Work out the finished part from the listing and answer in its coordinate system (mm). A direction names the side the tool comes from. Coordinates: 2 decimals unless noted, no trailing zeros. Order: outer loops, then holes, each group sorted by start corner. A loop starts at its lowest first (then second) coordinate and runs counter-clockwise, first axis right, second up. Notation, with made-up numbers: M 14,-11.5 L 29,-11.5 A15 cw 29,-6.5 Z; hole C -8.75,37.5 d4. An arc over 180 degrees is marked long. Write item = value, one per line. Start each with the question number.
Q1. Find section B-B on x = 20. Give the vertices of the cut face in (y, z), and give its area (3 significant figures).
Q2. A tool of negligible diameter and unlimited length cuts with its end or side. For faces 1 (the flat face through (-45.422, -23, 29)), 2 (the cylindrical face through (17.07, 13.09, 30.12)), from which of +Z, -Z, +X, -X, +Y, -Y can it reach the whole face along a straight path? Write none if from no direction.
Q3. Each of these flat-tipped pins is pushed along its axis until it touches: P1, Ø4, axis at x = -23.5, z = 32, coming from the +Y side; P2, Ø16.5, axis at x = 0, y = 0, coming from the +Z side; P3, Ø6, axis at y = -0.5, z = 34.5, coming from the -X side. Where does it stop, or does it pass through?
Q4. Straight lines are drawn through the part: line 1 along Y through (x, z) = (0, 1); line 2 along Y through (x, z) = (0, 15.5); line 3 along Z through (x, y) = (-19, -7.5). For each, find the intervals that lie inside material, in ascending order.
Q5. Find section C-C on x = -8. Give the vertices of the cut face in (y, z), and give its area (3 significant figures).
Q6. Determine the mould class of faces 3 (the flat face through (45.422, -23, 29)), 4 (the flat face through (-1, -24.666, 29)), 5 (the flat face through (-4, 4, 3)) for opening direction X: released by +X, released by -X, zero draft, split by the parting line, or undercut.
Q7. Find section A-A on y = 3.5. Give the vertices of the cut face in (x, z), and give its area (3 significant figures).
```python
from build123d import *

# Parameters (mm, degrees)
SKETCH1_R           = 24.241475666
SKETCH1_R_2         = 21.51
BOSS_EXTRUDE1_DEPTH = 58
SKETCH1_4_R         = 21.51
BOSS_EXTRUDE2_DEPTH = 3


with BuildPart() as part:
    # Sketch1 → Boss-Extrude1 (new body)
    # profile 1 of 2: a face of its own
    with BuildSketch(Plane.XY):
        Circle(SKETCH1_R)
        with Locations(Location((0, 0, 0), (0, 0, 180))):
            Circle(SKETCH1_R_2, mode=Mode.SUBTRACT)
    # profile 2 of 2: a face of its own
    with BuildSketch(Plane.XY):
        with BuildLine():
            Line((-45.421940828, -20.666245921), (-45.421940828, -24.666245921))
            Line((-45.421940828, -24.666245921), (45.421940828, -24.666245921))
            Line((45.421940828, -24.666245921), (45.421940828, -20.666245921))
            add(Edge.make_bspline(
                [(45.421940828, -20.666245921), (21.532203305, -20.666245921), (24.241475666, -19.078845964), (24.241475666, 0)],
                knots=[0, 0, 0, 0, 1, 1, 1, 1], degree=3))
            ThreePointArc((24.241475666, 0), (0, -24.241475666), (-24.241475666, 0))
            add(Edge.make_bspline(
                [(-45.421940828, -20.666245921), (-21.532203305, -20.666245921), (-24.241475666, -19.078845964), (-24.241475666, 0)],
                knots=[0, 0, 0, 0, 1, 1, 1, 1], degree=3))
        make_face()
    extrude(amount=BOSS_EXTRUDE1_DEPTH)

    # Sketch1_4 → Boss-Extrude2 (add)
    with BuildSketch(Plane.XY):
        with Locations(Location((0, 0, 0), (0, 0, 180))):
            Circle(SKETCH1_4_R)
        with BuildLine():
            ThreePointArc((0, -5.15), (-3.641599923, 3.641599923), (5.15, 0))
            ThreePointArc((5.15, 0), (3.641599923, -3.641599923), (0, -5.15))
        make_face(mode=Mode.SUBTRACT)
    extrude(amount=BOSS_EXTRUDE2_DEPTH)


solid = part.part
```
Findings below:
q1.outline = M -24.67,0 L 13.7,0 L 13.7,58 L 7.92,58 L 7.92,3 L -7.92,3 L -7.92,58 L -24.67,58 Z
q1.area = 1,350 mm^2
q2.face_1 = +Z, -Z, -X, +Y, -Y
q2.face_2 = +Z
q3.P1 = 11.2
q3.P2 = 3
q3.P3 = -24.24
q4.line_1 = -24.67 to -5.15, 5.15 to 24.24
q4.line_2 = -24.67 to -21.51, 21.51 to 24.24
q4.line_3 = 0 to 3
q5.outline = M -24.67,0 L 22.88,0 L 22.88,58 L 19.97,58 L 19.97,3 L -19.97,3 L -19.97,58 L -24.67,58 Z
q5.area = 562 mm^2
q6.face_3 = released by +X
q6.face_4 = zero draft
q6.face_5 = undercut
q7.outline = M -23.99,0 L -3.78,0 L -3.78,3 L -21.22,3 L -21.22,58 L -23.99,58 Z; M 3.78,0 L 23.99,0 L 23.99,58 L 21.22,58 L 21.22,3 L 3.78,3 Z
q7.area = 425 mm^2
